The listing builds one solid part. Answer for the finished solid, in the listing's coordinates (mm). Face numbers are marked on the shaded views. A direction names the side the tool comes from. Coordinates: 2 decimals unless noted, no trailing zeros. Write each loop counter-clockwise with the first axis right and the second up, starting at its lowest first coordinate (ties: lowest second). Pieces come first, ordered by that corner, then holes.
from build123d import *

# Parameters (mm, degrees)
SKETCH_R        = 7.5
PAD_DEPTH       = 2.5
SKETCH001_R     = 9.5
PAD001_DEPTH    = 1.5
SKETCH002_R     = 5.25
POCKET_DEPTH    = 2.5
SKETCH003_R     = 2.75
POCKET001_DEPTH = 5
CHAMFER_SIZE    = 1
CHAMFER001_SIZE = 1


with BuildPart() as part:
    # Sketch → Pad (new body)
    with BuildSketch(Plane.XY):
        Circle(SKETCH_R)
    extrude(amount=PAD_DEPTH)

    # Sketch001 (on Face3 of Pad) → Pad001 (join)
    with BuildSketch(Plane.XY.offset(2.5)):
        Circle(SKETCH001_R)
    extrude(amount=PAD001_DEPTH)

    # Sketch002 (on Face5 of Pad001) → Pocket (cut)
    with BuildSketch(Plane.XY.offset(4)):
        Circle(SKETCH002_R)
    extrude(amount=-POCKET_DEPTH, mode=Mode.SUBTRACT)

    # Sketch003 (on Face2 of Pocket) → Pocket001 (cut)
    with BuildSketch(Plane(origin=(0, 0, 0), x_dir=(1, 0, 0), z_dir=(0, 0, -1))):
        Circle(SKETCH003_R)
    extrude(amount=-POCKET001_DEPTH, mode=Mode.SUBTRACT)

    # Chamfer
    chamfer_edges = [part.edges().sort_by_distance(p)[0] for p in [
        (-9.5, 0, 4),
    ]]
    chamfer(chamfer_edges, length=CHAMFER_SIZE)

    # Chamfer001
    chamfer001_edges = [part.edges().sort_by_distance(p)[0] for p in [
        (-7.5, 0, 0),
    ]]
    chamfer(chamfer001_edges, length=CHAMFER001_SIZE)


solid = part.part
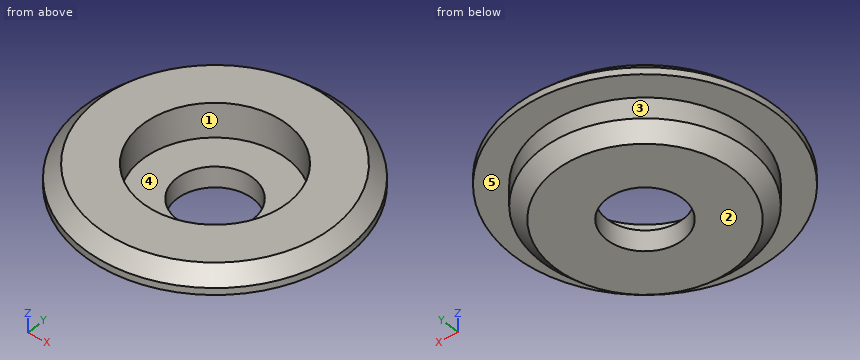
1. Find the intervals of material crossed by L1, parallel to Y at x = 0, z = 2.2; L2, parallel to Z at x = 6.75, y = -4.75; L3, parallel to Z at x = -2, y = -2, in increasing order.
Results found:
L1: y = -7.5 to -5.25, 5.25 to 7.5
L2: z = 2.5 to 4
L3: z = 0 to 1.5
2. Section C-C on z = 1.8 is taken. Give the vertices of the cut face in (x, y), then the cut area to 3 significant figures.
Results found:
outline: circle Ø15 at (0, 0); hole circle Ø10.5 at (0, 0)
area: 90.1 mm2
3. Section A-A on y = 0 is taken. Give the vertices of the cut face in (x, z), then the cut area to 3 significant figures.
Results found:
outline: (-9.5, 2.5) - (-7.5, 2.5) - (-7.5, 1) - (-6.5, 0) - (-2.75, 0) - (-2.75, 1.5) - (-5.25, 1.5) - (-5.25, 4) - (-8.5, 4) - (-9.5, 3) - close; (2.75, 0) - (6.5, 0) - (7.5, 1) - (7.5, 2.5) - (9.5, 2.5) - (9.5, 3) - (8.5, 4) - (5.25, 4) - (5.25, 1.5) - (2.75, 1.5) - close
area: 29.5 mm2
4. For a pull along Y with two mould halves and no side action, classify the marked faces 3, 4 and 5 as pulls with the +Y half, pulls with the -Y half, needs draft (parallel to the pull), parting line crosses it, or undercut.
Results found:
face 3: parting line crosses it
face 4: undercut
face 5: needs draft
5. Flat-ended cylindrical pins translate along their axes: P1, Ø1, axis at y = 6, z = 1, coming from the +X side; P2, Ø6.5, axis at x = 0, y = 0, coming from the -Z side; P3, Ø2, axis at y = 4, z = 2, coming from the +X side; P4, Ø1.5, axis at x = -2, z = 3.5, coming from the +Y side. Find the tip coordinate at first contact, or state that the pin passes through.
Results found:
P1: stops at x = 5.1
P2: stops at z = 0
P3: stops at x = 8.97
P4: stops at y = 9.39
6. A tool of negligible diameter and unlimited length cuts with its end or side. For the marked faces 1 and 2, from which of +Z, -Z, +X, -X, +Y, -Y can it reach the whole face along a straight path? Write none if from no direction.
Results found:
face 1: +Z
face 2: -Z, +X, -X, +Y, -Y
